```python
from build123d import *

# Parameters (mm, degrees)
SKETCH_1_R      = 60
SKETCH_1_R_2    = 3.3
EXTRUDE_1_DEPTH = 26
SKETCH_2_R      = 3.3
EXTRUDE_2_DEPTH = 36


with BuildPart() as part:
    # 草图1 → 凸台-拉伸1 (new body)
    with BuildSketch(Plane.XY.offset(6)):
        Circle(SKETCH_1_R)
        Circle(SKETCH_1_R_2, mode=Mode.SUBTRACT)
    extrude(amount=-EXTRUDE_1_DEPTH)

    # 草图2 → 凸台-拉伸2 (add)
    with BuildSketch(Plane(origin=(0, 0, -20), x_dir=(-1, 0, 0), z_dir=(0, 0, -1))):
        with Locations((-14.999999495, 40)):
            Circle(SKETCH_2_R)
        with Locations((14.999999495, 40)):
            Circle(SKETCH_2_R)
        with Locations((-14.999999495, -40)):
            Circle(SKETCH_2_R)
        with Locations((14.999999495, -40)):
            Circle(SKETCH_2_R)
    extrude(amount=-EXTRUDE_2_DEPTH)


solid = part.part
```
Read the model definition and answer for the solid it produces. Units are mm, in the model's axes. A direction names the side the tool comes from. Coordinates: 2 decimals unless noted, no trailing zeros. Loops run counter-clockwise (first coordinate to the right, second up) from the corner with the lowest first, then second, coordinate; pieces in that order, holes last. Notation, with made-up numbers: (30, -31.75) -> (79, -31.75) arc R21 cw to (79, -16.75) -> close; hole circle Ø8 at (34.5, 4.25). An arc over 180 degrees is marked (long way). Return JSON: item names as keys, results as strings.
Item 1: Find the intervals of material crossed by probe 1 along Y at (x, z) = (15, 9.5); probe 2 along Y at (x, z) = (0, -8.75); probe 3 along Z at (x, y) = (40, -20), in increasing order.
Answers:
{"probe 1": "y = -43.3 to -36.7, 36.7 to 43.3", "probe 2": "y = -60 to -3.3, 3.3 to 60", "probe 3": "z = -20 to 6"}
Item 2: For a pull along Y with two mould halves and no side action, classify faces 3 (the cylindrical face through (-2.43, 2.23, -6.82)), 4 (the flat face through (15, -40, 16)), 5 (the cylindrical face through (13.226, -37.217, 10.93)), 6 (the cylindrical face through (-59.94, 2.64, -6.82)) as +Y half, -Y half, draft (parallel to the pull), parting line (faces both ways), or undercut.
Answers:
{"face 3": "undercut", "face 4": "draft", "face 5": "undercut", "face 6": "parting line"}
Item 3: Find section A-A (x = 0). Determine the outline of the cut face in (y, z), plus the area to 3 significant figures.
Answers:
{"outline": "(-60, -20) -> (-3.3, -20) -> (-3.3, 6) -> (-60, 6) -> close; (3.3, -20) -> (60, -20) -> (60, 6) -> (3.3, 6) -> close", "area": "2,950 mm2"}
Item 4: Find section D-D (x = -15). Determine the outline of the cut face in (y, z).
Answers:
{"outline": "(-58.09, -20) -> (58.09, -20) -> (58.09, 6) -> (43.3, 6) -> (43.3, 16) -> (36.7, 16) -> (36.7, 6) -> (-36.7, 6) -> (-36.7, 16) -> (-43.3, 16) -> (-43.3, 6) -> (-58.09, 6) -> close"}
Item 5: Flat-ended cylindrical pins translate along their axes: P1, Ø6, axis at x = 27, z = -10, coming from the +Y side; P2, Ø6, axis at y = -35, z = -13.5, coming from the +X side; P3, Ø1.5, axis at x = -44, z = -14, coming from the -Y side; P4, Ø4, axis at x = 0, y = 0, coming from the -Z side. Find the tip coordinate at first contact, or state that the pin passes through.
Answers:
{"P1": "stops at y = 54.99", "P2": "stops at x = 50.75", "P3": "stops at y = -41.59", "P4": "passes through"}
Item 6: For faces 1 (the flat face through (-12, 1, -20)), 2 (the cylindrical face through (-16.774, -37.217, 10.93)), determine the directions among +Z, -Z, +X, -X, +Y, -Y from which every point of the face is accessible in a straight line to the end or side of a thin tool.
Answers:
{"face 1": "-Z, +X, -X, +Y, -Y", "face 2": "+Z"}
Item 7: Find section B-B (z = 14.5). Determine the outline of the cut face in (x, y), plus the area to 3 significant figures.
Answers:
{"outline": "circle Ø6.6 at (-15, -40); circle Ø6.6 at (-15, 40); circle Ø6.6 at (15, -40); circle Ø6.6 at (15, 40)", "area": "137 mm2"}
Item 8: Find section C-C (z = 3.5). Determine the outline of the cut face in (x, y).
Answers:
{"outline": "circle Ø120 at (0, 0); hole circle Ø6.6 at (0, 0)"}
